Autodesk Inventor part; units mm, degrees
ref_plane "YZ Plane" through (0, 0, 0) normal (1, 0, 0) x (0, 1, 0)
ref_plane "XZ Plane" through (0, 0, 0) normal (0, 1, 0) x (-1, 0, 0)
ref_plane "XY Plane" through (0, 0, 0) normal (0, 0, 1) x (1, 0, 0)
sketch "Sketch1" plane through (0, 0, 0) normal (0, 0, 1) x (1, 0, 0)
  line L0 (0, 0) -> (889, 0)
  line L1 (889, 0) -> (889, 38.1)
  line L2 (889, 38.1) -> (0, 38.1)
  line L3 (0, 38.1) -> (0, 0)
  dimension "d0" = 889
  dimension "d1" = 38.1
extrude "Extrusion1" add sketch "Sketch1" along normal blind 25.4
sketch "Sketch2" plane through (0, 0, 25.4) normal (0, 0, 1) x (1, 0, 0)
  line L0 (0, 38.1) -> (0, 0)
  line L1 (0, 0) -> (38.1, 0)
  line L2 (38.1, 0) -> (38.1, 38.1)
  line L3 (38.1, 38.1) -> (0, 38.1)
  line L4 (0, 38.1) -> (0, 0)
  line L5 (0, 0) -> (889, 0)
  line L6 (889, 0) -> (850.9, 0)
  line L7 (850.9, 0) -> (850.9, 38.1)
  line L8 (850.9, 38.1) -> (889, 38.1)
  line L9 (889, 38.1) -> (889, 0)
  dimension "d4" = 38.1
  dimension "d5" = 38.1
  dimension "d6" = 38.1
  dimension "d7" = 38.1
extrude "Extrusion2" cut sketch "Sketch2" against normal blind 12.7 contours L7 L8 L9 L5
sketch "Sketch5" plane through (0, 0, 25.4) normal (0, 0, 1) x (1, 0, 0)
  line L0 (0, 0) -> (38.1, 0)
  line L1 (38.1, 0) -> (38.1, 38.1)
  line L2 (38.1, 38.1) -> (0, 38.1)
  line L3 (0, 38.1) -> (0, 0)
  dimension "d10" = 38.1
  dimension "d11" = 38.1
extrude "Extrusion3" cut sketch "Sketch5" against normal blind 12.7
sketch "Sketch6" plane through (0, 0, 0) normal (0, -1, 0) x (1, 0, 0)
  line L0 (850.9, 12.7) -> (889, 12.7)
  line L1 (889, 12.7) -> (889, 9.525)
  line L2 (889, 0) -> (889, 12.7)
  line L3 (889, 9.525) -> (0, 9.525)
  line L4 (0, 9.525) -> (0, 15.875)
  line L5 (0, 15.875) -> (889, 15.875)
  line L6 (889, 15.875) -> (889, 12.7)
  dimension "d24" = 3.175
  dimension "d25" = 889
  dimension "d26" = 6.35
  dimension "d27" = 889
extrude "Extrusion4" cut sketch "Sketch6" against normal blind 6.35
properties part number "topv2" material "Wood (Cherry)"
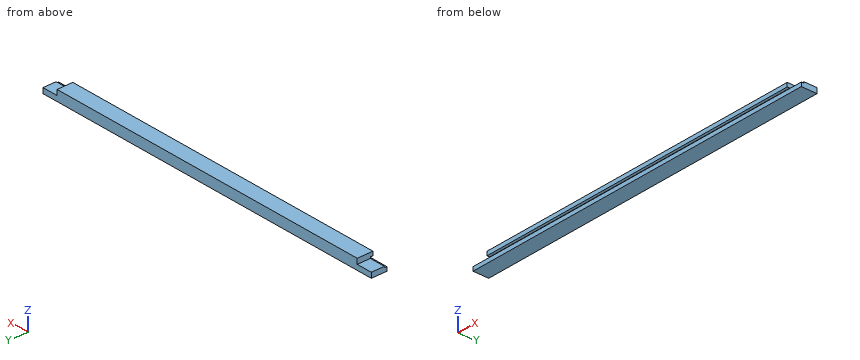
Part model, mm, in its own coordinate system. Coordinates: 2 decimals unless noted, no trailing zeros. Write each loop counter-clockwise with the first axis right and the second up, starting at its lowest first coordinate (ties: lowest second). Pieces come first, ordered by that corner, then holes.
Item 1: Slice it at A-A (x = 605). Write the cut outline in (y, z) (3 decimals), and give its area (3 significant figures).
Item 2: Pin check, flat tips, straight feed: pin 1 (4 mm diameter, centred on y = 18, z = 16.5, fed in from +X); pin 2 (1.9 mm diameter, centred on x = 655.5, z = 11.5, fed in from -Y); pin 3 (1 mm diameter, centred on y = 24, z = 20.5, fed in from -X). Stop position of each tip, or through.
Item 3: Slice it at C-C (z = 19.75). Write the cut outline in (x, y).
Item 4: Slice it at B-B (y = 14.5). Write the cut outline in (x, z).
Item 5: Probe line 1 (Z direction, x = 191, y = 6) (3 decimals); line 2 (Y direction, x = 354, z = 11); line 3 (X direction, y = 32, z = 20.25). List the from-to ranges inside material, lowest first.
Results found:
1. outline: (0, 0) - (38.1, 0) - (38.1, 25.4) - (0, 25.4) - (0, 15.875) - (6.35, 15.875) - (6.35, 9.525) - (0, 9.525) - close
1. area: 927 mm2
2. pin 1: stops at x = 850.9
2. pin 2: stops at y = 6.35
2. pin 3: stops at x = 38.1
3. outline: (38.1, 0) - (850.9, 0) - (850.9, 38.1) - (38.1, 38.1) - close
4. outline: (0, 0) - (889, 0) - (889, 12.7) - (850.9, 12.7) - (850.9, 25.4) - (38.1, 25.4) - (38.1, 12.7) - (0, 12.7) - close
5. line 1: z = 0 to 9.525, 15.875 to 25.4
5. line 2: y = 6.35 to 38.1
5. line 3: x = 38.1 to 850.9
